from build123d import *

# Parameters (mm, degrees)
F0_W     = 5
F0_H     = 20
F1_DEPTH = 60
F2_W     = 10
F2_H     = 35
F2_R     = 1.75
F2_W_2   = 20
F3_DEPTH = 5
F5_D     = 3
F5_DEPTH = 10
F5_TIP   = 0.9012909285


with BuildPart() as f1:
    # F0 (on Top) → F1 (new body)
    with BuildSketch(Plane.XY):
        Rectangle(F0_W, F0_H)
    extrude(amount=F1_DEPTH)

    # F2 (on face) → F3 (join)
    with BuildSketch(Plane.YZ.offset(2.5)):
        with Locations((15, 42.5)):
            Rectangle(F2_W, F2_H)
        with Locations((13.5, 28)):
            Circle(F2_R, mode=Mode.SUBTRACT)
        with Locations((13.5, 57)):
            Circle(F2_R, mode=Mode.SUBTRACT)
        with Locations((-15, 42.5)):
            Rectangle(F2_W, F2_H)
        with Locations((-13.5, 28)):
            Circle(F2_R, mode=Mode.SUBTRACT)
        with Locations((-13.5, 57)):
            Circle(F2_R, mode=Mode.SUBTRACT)
        with Locations((0, 42.5)):
            Rectangle(F2_W_2, F2_H)
    extrude(amount=F3_DEPTH)

    # F5
    with Locations(Plane(origin=(0, 0, 0), x_dir=(1, 0, 0), z_dir=(0, 0, -1))):
        with Locations((0, 0)):
            Hole(F5_D / 2, depth=F5_DEPTH)
            with Locations((0, 0, -(F5_DEPTH + F5_TIP / 2))):  # 118° drill point
                Cone(0, F5_D / 2, F5_TIP, mode=Mode.SUBTRACT)


solid = f1.part
Could you check a few things on this model? Use its own coordinates, in mm. A direction names the side the tool comes from. Give positions to 0.01 mm unless a question says otherwise; leave off trailing zeros. Order: outer loops, then holes, each group sorted by start corner. A loop starts at its lowest first (then second) coordinate and runs counter-clockwise, first axis right, second up.
Item 1: If we section it at C-C, the plane x = 6.5: Write out the boundary of the cut face in (y, z).
Item 2: If we mould it in two halves opening along Z, with no side actions, what happens to faces 5 (the face through (4.965, -11.831, 28.526)), 6 (the face through (5, 0, 25)), 7 (the face through (5, -20, 42))? For each: pulls with the +Z half, pulls with the -Z half, needs draft (parallel to the pull), parting line crosses it, or undercut.
Item 3: For faces 1 (the face through (2.5, -15, 43)), 2 (the face through (1.5, -0.07, 5.07)), 3 (the face through (2.5, 15, 43)), 4 (the face through (2.5, 0, 12)), which set-ups out of +Z, -Z, +X, -X, +Y, -Y let a thin tool reach every point of the face, with its end or its side?
Item 4: If we section it at D-D, the plane y = -6.5: Write out the boundary of the cut face in (x, z), plus the area to 3 significant figures.
Item 5: I need wall thicknesses on line 1 (Z direction, x = 5.35, y = -13.5); line 2 (X direction, y = -9, z = 22.5); line 3 (Y direction, x = 2, z = 55.5). Which ranges of each line are inside material? Lowest first, please.
Item 6: If we section it at B-B, the plane y = 13.5: Write out the boundary of the cut face in (x, z).
Item 7: I'm going to push flat-ended pins straight in: pin 1 (3 mm diameter, centred on y = 13.5, z = 28, fed in from -X); pin 2 (3 mm diameter, centred on y = 15, z = 40, fed in from -X); pin 3 (2.5 mm diameter, centred on x = 5, y = -4, fed in from -Z); pin 4 (5 mm diameter, centred on x = -1, y = 7, fed in from -Z). Where does each tip first touch, or does it pass through?
Item 8: If we section it at A-A, the plane z = 28: Write out the boundary of the cut face in (x, y), plus the area to 3 significant figures.
Values:
1. outline: (-20, 25) - (20, 25) - (20, 60) - (-20, 60) - close; hole circle Ø3.5 at (-13.5, 28); hole circle Ø3.5 at (-13.5, 57); hole circle Ø3.5 at (13.5, 28); hole circle Ø3.5 at (13.5, 57)
2. face 5: undercut
2. face 6: pulls with the -Z half
2. face 7: needs draft
3. face 1: +Z, -Z, -X, -Y
3. face 2: -Z
3. face 3: +Z, -Z, -X, +Y
3. face 4: -Z, +X, +Y, -Y
4. outline: (-2.5, 0) - (2.5, 0) - (2.5, 25) - (7.5, 25) - (7.5, 60) - (-2.5, 60) - close
4. area: 475 mm2
5. line 1: z = 25 to 26.25, 29.75 to 55.25, 58.75 to 60
5. line 2: x = -2.5 to 2.5
5. line 3: y = -10 to 10
6. outline: (2.5, 25) - (7.5, 25) - (7.5, 26.25) - (2.5, 26.25) - close; (2.5, 29.75) - (7.5, 29.75) - (7.5, 55.25) - (2.5, 55.25) - close; (2.5, 58.75) - (7.5, 58.75) - (7.5, 60) - (2.5, 60) - close
7. pin 1: passes through
7. pin 2: stops at x = 2.5
7. pin 3: stops at z = 25
7. pin 4: stops at z = 0
8. outline: (-2.5, -10) - (2.5, -10) - (2.5, -11.75) - (7.5, -11.75) - (7.5, 11.75) - (2.5, 11.75) - (2.5, 10) - (-2.5, 10) - close; (2.5, -20) - (7.5, -20) - (7.5, -15.25) - (2.5, -15.25) - close; (2.5, 15.25) - (7.5, 15.25) - (7.5, 20) - (2.5, 20) - close
8. area: 265 mm2
